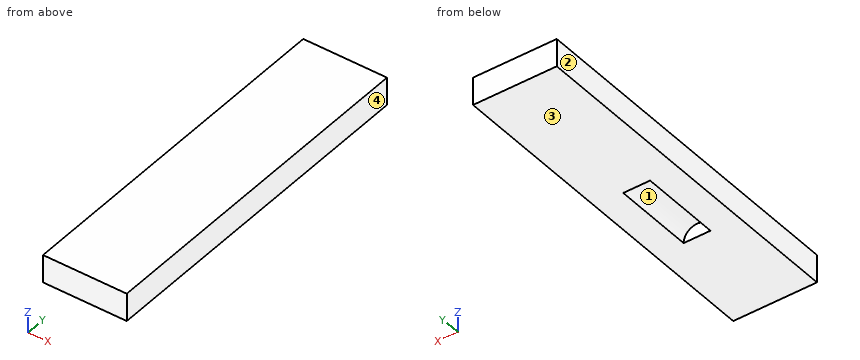
```python
from build123d import *

# Parameters (mm, degrees)
F0_W     = 12
F0_H     = 50
F0_W_2   = 1.925
F0_H_2   = 11.6
F1_DEPTH = 4
F2_ANGLE = 180


with BuildPart() as f1:
    # F0 (on Top) → F1 (new body)
    with BuildSketch(Plane.XY):
        Rectangle(F0_W, F0_H)
        Polygon((1.925, -10), (0, -10), (-1.925, -10), (-1.925, 1.6), (0, 1.6), (1.925, 1.6), align=None, mode=Mode.SUBTRACT)
        with Locations((-0.9625, -4.2)):
            Rectangle(F0_W_2, F0_H_2)
        with Locations((0.9625, -4.2)):
            Rectangle(F0_W_2, F0_H_2)
    extrude(amount=F1_DEPTH)

    # F0 (on Top) → F2 (revolve, cut)
    with BuildSketch(Plane.XY):
        with Locations((-0.9625, -4.2)):
            Rectangle(F0_W_2, F0_H_2)
    revolve(axis=Axis((0, -4.2, 0), (0, 1, 0)), revolution_arc=F2_ANGLE, mode=Mode.SUBTRACT)


solid = f1.part
```
Work out the finished part from the listing and answer in its coordinate system (mm). Face numbers are marked on the shaded views. Round coordinates to 2 decimals unless told otherwise and drop trailing zeros. Loops run counter-clockwise (first coordinate to the right, second up) from the corner with the lowest first, then second, coordinate; pieces in that order, holes last.
(1) Find the intervals of material crossed by L1, parallel to Y at x = 0.25, z = 1.35; L2, parallel to X at y = -5.5, z = 0.5; L3, parallel to Z at x = -1, y = -2.5, in increasing order.
Computed values:
L1: y = -25 to -10, 1.6 to 25
L2: x = -6 to -1.86, 1.86 to 6
L3: z = 1.64 to 4
(2) The mould has two halves that part along X. Classify the marked faces 1, 2, 3 and 4: pulls with the +X half, pulls with the -X half, needs draft (parallel to the pull), parting line crosses it, or undercut.
Computed values:
face 1: undercut
face 2: pulls with the -X half
face 3: needs draft
face 4: pulls with the +X half
(3) The part is cut by section C-C, the plane z = 1.2. Give the vertices of the cut face in (x, y), and give its area (3 significant figures).
Computed values:
outline: (-6, -25) - (6, -25) - (6, 25) - (-6, 25) - close; hole (-1.51, -10) - (1.51, -10) - (1.51, 1.6) - (-1.51, 1.6) - close
area: 565 mm2
(4) The part is cut by section A-A, the plane x = 0. Give the vertices of the cut face in (y, z) (3 decimals).
Computed values:
outline: (-25, 0) - (-10, 0) - (-10, 1.925) - (1.6, 1.925) - (1.6, 0) - (25, 0) - (25, 4) - (-25, 4) - close
(5) The part is cut by section B-B, the plane y = -6.5. Give the vertices of the cut face in (x, z) (3 decimals), and give its area (3 significant figures).
Computed values:
outline: (-6, 0) - (-1.925, 0) arc R1.925 cw to (1.925, 0) - (6, 0) - (6, 4) - (-6, 4) - close
area: 42.2 mm2
